Build history of the part. All positions in model axes, mm. Face numbers are marked on the shaded views. A direction names the side the tool comes from. Round coordinates to 2 decimals unless told otherwise and drop trailing zeros. Write each loop counter-clockwise with the first axis right and the second up, starting at its lowest first coordinate (ties: lowest second). Pieces come first, ordered by that corner, then holes. Notation, with made-up numbers: (-25.75, 24) - (30.25, 24) arc R9 ccw to (30.25, 38) - close; hole circle Ø1 at (68, 86.5). An arc over 180 degrees is marked (long way). Write each question's results on one line, items separated by ' | '.
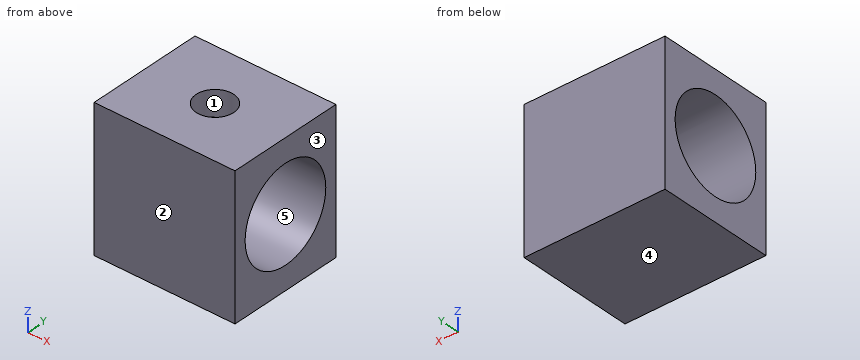
from build123d import *

# Parameters (mm, degrees)
SKETCH_1_W               = 30
SKETCH_1_H               = 25
EXTRUDE_1_DEPTH          = 15
SKETCH_3_R               = 10
CUT_EXTRUDE_1_DEPTH      = 36.794552658
CUT_EXTRUDE_2_REACH      = 37.795
CUT_EXTRUDE_2_END_RADIUS = 10
SKETCH_4_R               = 4


with BuildPart() as part:
    # 草图1 → 凸台-拉伸1 (new, symmetric)
    with BuildSketch(Plane.XY):
        Rectangle(SKETCH_1_W, SKETCH_1_H)
    extrude(amount=EXTRUDE_1_DEPTH, both=True)

    # 草图3 → 切除-拉伸1 (cut, through all)
    with BuildSketch(Plane.ZY.offset(15)):
        Circle(SKETCH_3_R)
    extrude(amount=-CUT_EXTRUDE_1_DEPTH, mode=Mode.SUBTRACT)

    # 切除-拉伸2: up to this cylinder (the profile starts outside it)
    cut_extrude_2_end = Plane(origin=(0, 0, 0), z_dir=(-1, 0, 0)) * Cylinder(CUT_EXTRUDE_2_END_RADIUS, 96.59, mode=Mode.PRIVATE)
    # 草图4 → 切除-拉伸2 (cut, up to the surface)
    with BuildSketch(Plane.XY.offset(15), mode=Mode.PRIVATE) as cut_extrude_2_sk1:
        Circle(SKETCH_4_R)
    cut_extrude_2_tool1 = extrude(cut_extrude_2_sk1.sketch, amount=-CUT_EXTRUDE_2_REACH, mode=Mode.PRIVATE) - cut_extrude_2_end
    add(cut_extrude_2_tool1.solids().sort_by_distance((0, 0, 15))[0], mode=Mode.SUBTRACT)


solid = part.part
(1) Slice it at D-D, the plane y = -5.5. Write the cut outline in (x, z), and give its area (3 significant figures).
Worked answers:
outline: (-15, -15) - (15, -15) - (15, -8.35) - (-15, -8.35) - close; (-15, 8.35) - (15, 8.35) - (15, 15) - (-15, 15) - close | area: 399 mm2
(2) Slice it at A-A, the plane y = 0. Write the cut outline in (x, z), and give its area (3 significant figures).
Worked answers:
outline: (-15, -15) - (15, -15) - (15, -10) - (-15, -10) - close; (-15, 10) - (-4, 10) - (-4, 15) - (-15, 15) - close; (4, 10) - (15, 10) - (15, 15) - (4, 15) - close | area: 260 mm2
(3) Flat gauge pin, fed straight in: pin 1 Ø1.5 at (x, y) = (-1, 0) entering from +Z. Where does the tip first touch, or does it go through?
Worked answers:
pin 1: stops at z = -9.97
(4) Tool access for the marked faces 1 and 2: list every direction of +Z, -Z, +X, -X, +Y, -Y with a clear straight run to the whole face (end or side of a thin tool).
Worked answers:
face 1: +Z | face 2: +Z, -Z, +X, -X, -Y
(5) Drill centre lines: probe 1 along Y at (x, z) = (3, 0); probe 2 along Y at (x, z) = (-6.5, -2.5); probe 3 along Z at (x, y) = (7, 8). Where is each one in solid material? Low to high. Write a range as [from, to].
Worked answers:
probe 1: y = [-12.5, -10], [10, 12.5] | probe 2: y = [-12.5, -9.68], [9.68, 12.5] | probe 3: z = [-15, -6], [6, 15]
(6) Slice it at C-C, the plane z = 11.5. Write the cut outline in (x, y).
Worked answers:
outline: (-15, -12.5) - (15, -12.5) - (15, 12.5) - (-15, 12.5) - close; hole circle Ø8 at (0, 0)
(7) Two-plate mould, pull along Z, no slides. Class the marked faces 3, 4 and 5: released by +Z, released by -Z, zero draft, split by the parting line, or undercut.
Worked answers:
face 3: zero draft | face 4: released by -Z | face 5: undercut
(8) Slice it at B-B, the plane z = 0. Write the cut outline in (x, y).
Worked answers:
outline: (-15, -12.5) - (15, -12.5) - (15, -10) - (-15, -10) - close; (-15, 10) - (15, 10) - (15, 12.5) - (-15, 12.5) - close
